Autodesk Inventor part; units mm, degrees
ref_plane "YZ Plane" through (0, 0, 0) normal (1, 0, 0) x (0, 1, 0)
ref_plane "XZ Plane" through (0, 0, 0) normal (0, 1, 0) x (-1, 0, 0)
ref_plane "XY Plane" through (0, 0, 0) normal (0, 0, 1) x (1, 0, 0)
sketch "Skizze1" plane through (0, 0, 0) normal (0, 0, 1) x (1, 0, 0)
  arc A0 (-10.6401, 53.1217) -> (-12.6401, 51.1217) centre (-10.6401, 51.1217) ccw construction
  line L0 (-12.6401, 51.1217) -> (-12.6401, -3.8783) construction
  arc A1 (-12.6401, -3.8783) -> (-10.6401, -5.8783) centre (-10.6401, -3.8783) ccw construction
  line L1 (-10.6401, -5.8783) -> (35.6599, -5.8783) construction
  arc A2 (35.6599, -5.8783) -> (37.6599, -3.8783) centre (35.6599, -3.8783) ccw construction
  line L2 (37.6599, -3.8783) -> (37.6599, 51.1217) construction
  arc A3 (37.6599, 51.1217) -> (35.6599, 53.1217) centre (35.6599, 51.1217) ccw construction
  line L3 (35.6599, 53.1217) -> (-10.6401, 53.1217) construction
  arc A4 (-24.2401, -8.4283) -> (-19.5401, -13.1283) centre (-19.5401, -8.4283) ccw construction
  line L4 (-24.2401, 55.6717) -> (-24.2401, -8.4283) construction
  arc A5 (-19.5401, 60.3717) -> (-24.2401, 55.6717) centre (-19.5401, 55.6717) ccw construction
  line L5 (44.5599, 60.3717) -> (-19.5401, 60.3717) construction
  arc A6 (49.2599, 55.6717) -> (44.5599, 60.3717) centre (44.5599, 55.6717) ccw construction
  line L6 (49.2599, -8.4283) -> (49.2599, 55.6717) construction
  arc A7 (44.5599, -13.1283) -> (49.2599, -8.4283) centre (44.5599, -8.4283) ccw construction
  line L7 (-19.5401, -13.1283) -> (44.5599, -13.1283) construction
  line L8 (35.6599, -5.7783) -> (-10.6401, -5.7783)
  arc A8 (-12.5401, -3.8783) -> (-10.6401, -5.7783) centre (-10.6401, -3.8783) ccw
  line L9 (-12.5401, -3.8783) -> (-12.5401, 51.1217)
  arc A9 (-10.6401, 53.0217) -> (-12.5401, 51.1217) centre (-10.6401, 51.1217) ccw
  line L10 (-10.6401, 53.0217) -> (35.6599, 53.0217)
  arc A10 (37.5599, 51.1217) -> (35.6599, 53.0217) centre (35.6599, 51.1217) ccw
  line L11 (37.5599, 51.1217) -> (37.5599, -3.8783)
  arc A11 (35.6599, -5.7783) -> (37.5599, -3.8783) centre (35.6599, -3.8783) ccw
  line L12 (12.5099, -5.7783) -> (12.5099, 53.0217) construction
  line L13 (12.3599, 53.0217) -> (12.3599, -5.7783)
  point P0 (0, 0)
  dimension "d0" = 0.1
  dimension "d1" = 24.9
extrude "Extrusion1" add sketch "Skizze1" along normal blind 1.8 contours L8 A8 L9 A9 L10 L13
sketch "Skizze2" plane through (0, 0, 1.8) normal (0, 0, 1) x (1, 0, 0)
  line L0 (12.3599, 56.5217) -> (-12.5401, 56.5217)
  line L1 (-12.5401, 56.5217) -> (-12.5401, -9.2783)
  line L2 (-12.5401, -9.2783) -> (12.3599, -9.2783)
  line L3 (12.3599, -9.2783) -> (12.3599, 56.5217)
  line L4 (-10.6401, -5.7783) -> (12.3599, -5.7783)
  line L5 (12.3599, 53.0217) -> (-10.6401, 53.0217)
  line L6 (12.3599, -5.7783) -> (12.3599, 53.0217)
  line L7 (-12.5401, 51.1217) -> (-12.5401, -3.8783)
  arc A0 (-0.5286, -10.1283) -> (-4.4516, -10.1283) centre (-2.4901, -8.5783) ccw
  arc A1 (-4.3683, 57.4717) -> (-0.612, 57.4717) centre (-2.4901, 55.8217) ccw
  circle A2 centre (-2.4901, -8.5783) radius 2.65 construction
  arc A3 (0.0658, -9.2783) -> (-5.046, -9.2783) centre (-2.4901, -8.5783) ccw
  circle A4 centre (-2.4901, 55.8217) radius 2.65 construction
  arc A5 (-5.046, 56.5217) -> (0.0658, 56.5217) centre (-2.4901, 55.8217) ccw
  point P0 (0, 0)
  dimension "d4" = 3.5
  dimension "d5" = 3.5
  dimension "d30" = 2.5
  dimension "d31" = 5.3
  dimension "d32" = 2.5
  dimension "d33" = 5.3
extrude "Extrusion2" add sketch "Skizze2" along normal blind 0.8 contours L3 L2 A3 L1 L0 A5
sketch "Skizze3" plane through (0, 0, 2.6) normal (0, 0, 1) x (1, 0, 0)
  line L0 (-11.5401, 51.0217) -> (6.4599, 51.0217)
  line L1 (6.4599, 51.0217) -> (6.4599, 44.0217)
  line L2 (6.4599, 44.0217) -> (-11.5401, 44.0217)
  line L3 (-11.5401, 44.0217) -> (-11.5401, 51.0217)
  line L4 (-11.5401, 3.2217) -> (6.4599, 3.2217)
  line L5 (6.4599, 3.2217) -> (6.4599, -3.7783)
  line L6 (6.4599, -3.7783) -> (-11.5401, -3.7783)
  line L7 (-11.5401, -3.7783) -> (-11.5401, 3.2217)
  line L8 (12.3599, 56.5217) -> (-12.5401, 56.5217)
  line L9 (-12.5401, -9.2783) -> (12.3599, -9.2783)
  line L10 (-12.5401, -3.8783) -> (-12.5401, -9.2783)
  point P0 (0, 0)
  dimension "d8" = 18
  dimension "d9" = 18
  dimension "d10" = 7
  dimension "d11" = 7
  dimension "d12" = 5.5
  dimension "d13" = 5.5
  dimension "d14" = 1
extrude "Extrusion3" add sketch "Skizze3" along normal blind 0.4
chamfer "Fase1" distance 1 angle 45 5 edges at (0.8599, 53.0217, 0) (-11.9836, 52.4652, 0) (-12.5401, 23.6217, 0) (-11.9836, -5.2218, 0) (0.8599, -5.7783, 0)
sketch "Skizze4" plane through (0, 0, 0) normal (0, 0, -1) x (-1, 0, 0)
  line L0 (10.6401, -4.7783) -> (-12.3599, -4.7783) construction
  line L1 (-12.3599, 52.0217) -> (10.6401, 52.0217) construction
  line L2 (-6.9071, 11.4129) -> (4.4149, 11.4129) construction
  line L3 (4.4149, 11.4129) -> (4.4149, 1.8512) construction
  line L4 (4.4149, 1.8512) -> (-6.9071, 1.8512) construction
  line L5 (-6.9071, 1.8512) -> (-6.9071, 11.4129) construction
  line L6 (-3.8878, 41.1888) -> (4.1122, 41.1888) construction
  line L7 (4.1122, 41.1888) -> (4.1122, 36.9997) construction
  line L8 (4.1122, 36.9997) -> (-3.8878, 36.9997) construction
  line L9 (-3.8878, 36.9997) -> (-3.8878, 41.1888) construction
  line L10 (11.5401, 51.1217) -> (11.5401, -3.8783) construction
  line L11 (11.5401, 40.0217) -> (-12.3599, 40.0217) construction
  line L12 (11.5401, 7.2217) -> (-12.3599, 7.2217) construction
  line L13 (-12.3599, -4.7783) -> (-12.3599, 52.0217) construction
  line L14 (-0.8599, -4.7783) -> (-0.8599, 52.0217) construction
  line L15 (3.8385, 6.0547) -> (-0.2263, 6.0547)
  line L16 (-0.2263, 6.0547) -> (-0.2263, 1.9899)
  line L17 (-0.2263, 1.9899) -> (-1.5683, 1.9899)
  line L18 (-1.5683, 1.9899) -> (-1.5683, 6.0547)
  line L19 (-1.5683, 6.0547) -> (-5.6332, 6.0547)
  line L20 (-5.6332, 6.0547) -> (-5.6332, 7.348)
  line L21 (-5.6332, 7.348) -> (-1.5683, 7.348)
  line L22 (-1.5683, 7.348) -> (-1.5683, 11.4129)
  line L23 (-1.5683, 11.4129) -> (-0.2263, 11.4129)
  line L24 (-0.2263, 11.4129) -> (-0.2263, 7.348)
  line L25 (-0.2263, 7.348) -> (3.8385, 7.348)
  line L26 (3.8385, 7.348) -> (3.8385, 6.0547)
  line L27 (1.3829, 39.7301) -> (-3.1585, 39.7301)
  line L28 (-3.1585, 39.7301) -> (-3.1585, 41.1888)
  line L29 (-3.1585, 41.1888) -> (1.3829, 41.1888)
  line L30 (1.3829, 41.1888) -> (1.3829, 39.7301)
  point P0 (0, 0)
  dimension "d20" = 12
  dimension "d21" = 12
extrude "Extrusion4" cut sketch "Skizze4" against normal blind 0.4
sketch "Skizze5" plane through (0, 0, 2.6) normal (0, 0, 1) x (1, 0, 0)
  line L0 (7.3599, 32.0217) -> (-7.5401, 32.0217)
  line L1 (-7.5401, 32.0217) -> (-7.5401, 15.2217)
  line L2 (-7.5401, 15.2217) -> (7.3599, 15.2217)
  line L3 (7.3599, 15.2217) -> (7.3599, 32.0217)
  line L4 (6.4599, 44.0217) -> (-11.5401, 44.0217)
  line L5 (6.4599, 3.2217) -> (-11.5401, 3.2217)
  line L6 (-12.5401, 56.5217) -> (-12.5401, -9.2783)
  line L7 (12.3599, -9.2783) -> (12.3599, 56.5217)
  point P0 (0, 0)
  dimension "d24" = 12
  dimension "d25" = 12
  dimension "d26" = 5
  dimension "d27" = 5
extrude "Extrusion5" cut sketch "Skizze5" against normal blind 0.6
equation "\"d5\" = d4"
equation "\"d9\" = d8"
equation "\"d13\" = d12"
properties part number "Button"
Verification items for the finished model (mm, model axes). A direction names the side the tool comes from. Coordinates: 2 decimals unless noted, no trailing zeros. Loops run counter-clockwise (first coordinate to the right, second up) from the corner with the lowest first, then second, coordinate; pieces in that order, holes last. Notation, with made-up numbers: (42, -36.75) -> (85, -36.75) arc R9 ccw to (85, -19.75) -> close; hole circle Ø10 at (-28.75, 30.25). An arc over 180 degrees is marked (long way). Write each question's results on one line, items separated by ' | '.
Item 1: Material ranges on L1, parallel to X at y = 21.5, z = 2.5; L2, parallel to Y at x = 0.5, z = 2.4; L3, parallel to Z at x = -9.5, y = 30, recorded low to high.
Found:
L1: x = -12.54 to -7.54, 7.36 to 12.36 | L2: y = -9.28 to 15.22, 32.02 to 56.52 | L3: z = 0 to 2.6
Item 2: Gauge pin test, flat ends, axial feed: pin 1 (5 mm diameter, centred on x = -2.49, y = -8.58, fed in from -Z); pin 2 (6 mm diameter, centred on x = 4.5, y = 24, fed in from +Z). Record the tip position at first contact, or that the pin passes through.
Found:
pin 1: passes through | pin 2: stops at z = 2.6
Item 3: Section check C-C, the plane y = -1. Enter the section's corners in (x, z), plus the area to 3 significant figures.
Found:
outline: (-12.54, 1) -> (-11.54, 0) -> (12.36, 0) -> (12.36, 2.6) -> (6.46, 2.6) -> (6.46, 3) -> (-11.54, 3) -> (-11.54, 2.6) -> (-12.54, 2.6) -> close | area: 71.4 mm2
Item 4: Section check A-A, the plane x = 8.5. Enter the section's corners in (y, z), plus the area to 3 significant figures.
Found:
outline: (-9.28, 1.8) -> (-5.78, 1.8) -> (-5.78, 1) -> (-4.78, 0) -> (52.02, 0) -> (53.02, 1) -> (53.02, 1.8) -> (56.52, 1.8) -> (56.52, 2.6) -> (-9.28, 2.6) -> close | area: 157 mm2
Item 5: Section check B-B, the plane y = 40.5. Enter the section's corners in (x, z).
Found:
outline: (-12.54, 1) -> (-11.54, 0) -> (-1.38, 0) -> (-1.38, 0.4) -> (3.16, 0.4) -> (3.16, 0) -> (12.36, 0) -> (12.36, 2.6) -> (-12.54, 2.6) -> close
Item 6: Tool access check on faces 1 (the face through (1, 40, 0.4)), 2 (the face through (-12, 52.45, 1.39)), 3 (the face through (0, 24, 2)), 4 (the face through (-11.969, -5.236, 1.394)). Record the directions out of +Z, -Z, +X, -X, +Y, -Y that give a thin tool (end or side, any length) a straight path to the whole face; none if there is none.
Found:
face 1: -Z | face 2: -Z, -X, +Y | face 3: +Z | face 4: -Z, -X, -Y
Item 7: Mould release check, pull along X, two halves, no side actions. Record for faces 5 (the face through (12.36, 24, 1)), 6 (the face through (1, 7, 0.4)), 7 (the face through (-11.55, 52.05, 0.4)): +X half, -X half, draft (parallel to the pull), parting line (faces both ways), or undercut.
Found:
face 5: +X half | face 6: undercut | face 7: -X half
